Build history of the part. All positions in model axes, mm. A direction names the side the tool comes from. Give positions to 0.01 mm unless a question says otherwise; leave off trailing zeros. Loops run counter-clockwise (first coordinate to the right, second up) from the corner with the lowest first, then second, coordinate; pieces in that order, holes last.
1) Band-saw the part on C-C on x = 19. List the corners of the cut face in (y, z).
2) Band-saw the part on D-D on y = 39. List the corners of the cut face in (x, z), then the cut area to 3 significant figures.
3) 3-axis set-ups, long thin cutter, end or side, ignore diameter. For faces 1 (the flat face through (-21, 10, 0)), 2 (the flat face through (0, 21, 0)), 3 (the flat face through (-4.93, 28.9, -8.7)), 4 (the flat face through (-10, 29, 0)): which of +Z, -Z, +X, -X, +Y, -Y reach the whole face in a straight line?
4) Wall check: line 1 (X direction, y = 12.3, z = -20); line 2 (X direction, y = 13, z = 0). Give the ranges that are in metal, low to high.
5) Band-saw the part on B-B on z = 0. List the corners of the cut face in (x, y), then the cut area to 3 significant figures.
6) Flat gauge pins, fed straight in: P1, Ø1.5, axis at x = -4, y = 24, coming from the -Z side; P2, Ø22.5, axis at x = 5, z = 4.5, coming from the -Y side; P3, Ø3, axis at y = 40.5, z = -6.5, coming from the -X side (3 decimals); P4, Ø3, axis at y = 40.5, z = 10, coming from the -X side. Where does each tip first touch, or does it go through?
7) Band-saw the part on A-A on y = 5.5. List the corners of the cut face in (x, z), then the cut area to 3 significant figures.
8) Two-plate mould, pull along Z, no slides. Class faces 5 (the flat face through (0, 10, 21)), 6 (the cylindrical face through (-26.68, 4.93, -0.3)), 7 (the cylindrical face through (-25.68, 4.44, -0.29)): +Z half, -Z half, draft (parallel to the pull), parting line (faces both ways), or undercut.
```python
from build123d import *

# Parameters (mm, degrees)
SKETCH3_R             = 4
BOSS_EXTRUDE2_DEPTH   = 10
SKETCH4_R             = 15
BOSS_EXTRUDE3_DEPTH   = 12
SHELL2_T              = -1
BOSS_EXTRUDE4_DEPTH   = 14
SKETCH6_R             = 8
BOSS_EXTRUDE5_DEPTH   = 12
BOSS_EXTRUDE6_DEPTH   = 5
M5X0_8_TAPPED_HOLE1_D = 4.2


with BuildPart() as part:
    # Sketch3 → Boss-Extrude2 (new body)
    with BuildSketch(Plane(origin=(0, 0, 0), x_dir=(1, 0, 0), z_dir=(0, 1, 0))):
        with Locations((-20, -20)):
            Circle(SKETCH3_R)
        with BuildLine():
            ThreePointArc((23.859011112, 21.052631579), (23.964596098, 20.531015797), (24, 20))
            ThreePointArc((24, 20), (16.821122343, 17.572092085), (21.052631579, 23.859011112))
            ThreePointArc((21.052631579, 23.859011112), (0, 26.678788881), (-21.052631579, 23.859011112))
            ThreePointArc((-21.052631579, 23.859011112), (-17.572092085, 23.178877657), (-16, 20))
            ThreePointArc((-16, 20), (-20.531015797, 16.035403902), (-23.859011112, 21.052631579))
            ThreePointArc((-23.859011112, 21.052631579), (-26.678788881, 0), (-23.859011112, -21.052631579))
            ThreePointArc((-23.859011112, -21.052631579), (-20.531015797, -16.035403902), (-16, -20))
            ThreePointArc((-16, -20), (-17.572092085, -23.178877657), (-21.052631579, -23.859011112))
            ThreePointArc((-21.052631579, -23.859011112), (0, -26.678788881), (21.052631579, -23.859011112))
            ThreePointArc((21.052631579, -23.859011112), (16.821122343, -17.572092085), (24, -20))
            ThreePointArc((24, -20), (23.964596098, -20.531015797), (23.859011112, -21.052631579))
            ThreePointArc((23.859011112, -21.052631579), (26.678788881, 0), (23.859011112, 21.052631579))
        make_face()
        with Locations((-20, 20)):
            Circle(SKETCH3_R)
        with Locations((20, -20)):
            Circle(SKETCH3_R)
        with Locations((20, 20)):
            Circle(SKETCH3_R)
    extrude(amount=BOSS_EXTRUDE2_DEPTH)

    # Sketch4 → Boss-Extrude3 (add)
    with BuildSketch(Plane(origin=(0, 10, 0), x_dir=(1, 0, 0), z_dir=(0, 1, 0))):
        with Locations(Location((0, 0, 0), (0, 0, 270))):
            Circle(SKETCH4_R)
    extrude(amount=BOSS_EXTRUDE3_DEPTH)

    # Shell2
    shell2_openings = [part.faces().sort_by_distance(p)[0] for p in [
        (0, 0, 0),
    ]]
    offset(amount=SHELL2_T, openings=shell2_openings, kind=Kind.INTERSECTION)

    # Sketch5 → Boss-Extrude4 (add)
    with BuildSketch(Plane(origin=(0, 22, 0), x_dir=(1, 0, 0), z_dir=(0, 1, 0))):
        Polygon((0, 11.547005384), (-10, 5.773502692), (-10, -5.773502692), (0, -11.547005384), (10, -5.773502692), (10, 5.773502692), align=None)
    extrude(amount=BOSS_EXTRUDE4_DEPTH)

    # Sketch6 → Boss-Extrude5 (add)
    with BuildSketch(Plane(origin=(0, 36, 0), x_dir=(1, 0, 0), z_dir=(0, 1, 0))):
        with Locations(Location((0, 0, 0), (0, 0, 270))):
            Circle(SKETCH6_R)
    extrude(amount=BOSS_EXTRUDE5_DEPTH)

    # Sketch7 → Boss-Extrude6 (add)
    with BuildSketch(Plane(origin=(0, 10, 0), x_dir=(1, 0, 0), z_dir=(0, 1, 0))):
        with BuildLine():
            ThreePointArc((23.859011112, 21.052631579), (22.828427125, 22.828427125), (21.052631579, 23.859011112))
            ThreePointArc((21.052631579, 23.859011112), (18.973409384, 23.866020138), (17.171572875, 22.828427125))
            ThreePointArc((17.171572875, 22.828427125), (16.30448187, 21.530733729), (16, 20))
            Line((16, 20), (20, 20))
            Line((20, 20), (20, 16))
            ThreePointArc((20, 16), (21.530733729, 16.30448187), (22.828427125, 17.171572875))
            ThreePointArc((22.828427125, 17.171572875), (23.69551813, 18.469266271), (24, 20))
            ThreePointArc((24, 20), (23.964596098, 20.531015797), (23.859011112, 21.052631579))
        make_face()
        with BuildLine():
            Line((20, 20), (16, 20))
            ThreePointArc((16, 20), (16.30448187, 18.469266271), (17.171572875, 17.171572875))
            Line((17.171572875, 17.171572875), (20, 20))
        make_face()
        with BuildLine():
            Line((20, 16), (20, 20))
            Line((20, 20), (17.171572875, 17.171572875))
            ThreePointArc((17.171572875, 17.171572875), (18.469266271, 16.30448187), (20, 16))
        make_face()
        with BuildLine():
            Line((17.171572875, 17.171572875), (10.606601718, 10.606601718))
            ThreePointArc((10.606601718, 10.606601718), (11.937336386, 9.082951062), (13.050951275, 7.394097025))
            Line((13.050951275, 7.394097025), (20, 14.343145751))
            Line((20, 14.343145751), (20, 16))
            ThreePointArc((20, 16), (18.469266271, 16.30448187), (17.171572875, 17.171572875))
        make_face()
        with BuildLine():
            Line((16, 20), (14.343145751, 20))
            Line((14.343145751, 20), (7.394097025, 13.050951275))
            ThreePointArc((7.394097025, 13.050951275), (9.082951062, 11.937336386), (10.606601718, 10.606601718))
            Line((10.606601718, 10.606601718), (17.171572875, 17.171572875))
            ThreePointArc((17.171572875, 17.171572875), (16.30448187, 18.469266271), (16, 20))
        make_face()
        with BuildLine():
            ThreePointArc((-7.394097025, -13.050951275), (-9.082951062, -11.937336386), (-10.606601718, -10.606601718))
            Line((-10.606601718, -10.606601718), (-17.171572875, -17.171572875))
            ThreePointArc((-17.171572875, -17.171572875), (-16.30448187, -18.469266271), (-16, -20))
            Line((-16, -20), (-14.343145751, -20))
            Line((-14.343145751, -20), (-7.394097025, -13.050951275))
        make_face()
        with BuildLine():
            Line((-17.171572875, -17.171572875), (-10.606601718, -10.606601718))
            ThreePointArc((-10.606601718, -10.606601718), (-11.937336386, -9.082951062), (-13.050951275, -7.394097025))
            Line((-13.050951275, -7.394097025), (-20, -14.343145751))
            Line((-20, -14.343145751), (-20, -16))
            ThreePointArc((-20, -16), (-18.469266271, -16.30448187), (-17.171572875, -17.171572875))
        make_face()
        with BuildLine():
            ThreePointArc((-16, -20), (-16.30448187, -18.469266271), (-17.171572875, -17.171572875))
            Line((-17.171572875, -17.171572875), (-20, -20))
            Line((-20, -20), (-16, -20))
        make_face()
        with BuildLine():
            Line((-20, -20), (-17.171572875, -17.171572875))
            ThreePointArc((-17.171572875, -17.171572875), (-18.469266271, -16.30448187), (-20, -16))
            Line((-20, -16), (-20, -20))
        make_face()
        with BuildLine():
            ThreePointArc((-22.828427125, -17.171572875), (-23.866020138, -18.973409384), (-23.859011112, -21.052631579))
            ThreePointArc((-23.859011112, -21.052631579), (-22.828427125, -22.828427125), (-21.052631579, -23.859011112))
            ThreePointArc((-21.052631579, -23.859011112), (-18.973409384, -23.866020138), (-17.171572875, -22.828427125))
            ThreePointArc((-17.171572875, -22.828427125), (-16.30448187, -21.530733729), (-16, -20))
            Line((-16, -20), (-20, -20))
            Line((-20, -20), (-20, -16))
            ThreePointArc((-20, -16), (-21.530733729, -16.30448187), (-22.828427125, -17.171572875))
        make_face()
        with BuildLine():
            ThreePointArc((21.052631579, -23.859011112), (22.828427125, -22.828427125), (23.859011112, -21.052631579))
            ThreePointArc((23.859011112, -21.052631579), (23.964596098, -20.531015797), (24, -20))
            ThreePointArc((24, -20), (23.69551813, -18.469266271), (22.828427125, -17.171572875))
            ThreePointArc((22.828427125, -17.171572875), (21.530733729, -16.30448187), (20, -16))
            Line((20, -16), (20, -20))
            Line((20, -20), (16, -20))
            ThreePointArc((16, -20), (16.30448187, -21.530733729), (17.171572875, -22.828427125))
            ThreePointArc((17.171572875, -22.828427125), (18.973409384, -23.866020138), (21.052631579, -23.859011112))
        make_face()
        with BuildLine():
            Line((20, -20), (17.171572875, -17.171572875))
            ThreePointArc((17.171572875, -17.171572875), (16.30448187, -18.469266271), (16, -20))
            Line((16, -20), (20, -20))
        make_face()
        with BuildLine():
            ThreePointArc((20, -16), (18.469266271, -16.30448187), (17.171572875, -17.171572875))
            Line((17.171572875, -17.171572875), (20, -20))
            Line((20, -20), (20, -16))
        make_face()
        with BuildLine():
            ThreePointArc((13.050951275, -7.394097025), (11.937336386, -9.082951062), (10.606601718, -10.606601718))
            Line((10.606601718, -10.606601718), (17.171572875, -17.171572875))
            ThreePointArc((17.171572875, -17.171572875), (18.469266271, -16.30448187), (20, -16))
            Line((20, -16), (20, -14.343145751))
            Line((20, -14.343145751), (13.050951275, -7.394097025))
        make_face()
        with BuildLine():
            Line((17.171572875, -17.171572875), (10.606601718, -10.606601718))
            ThreePointArc((10.606601718, -10.606601718), (9.082951062, -11.937336386), (7.394097025, -13.050951275))
            Line((7.394097025, -13.050951275), (14.343145751, -20))
            Line((14.343145751, -20), (16, -20))
            ThreePointArc((16, -20), (16.30448187, -18.469266271), (17.171572875, -17.171572875))
        make_face()
        with BuildLine():
            Line((17.171572875, 22.828427125), (14.343145751, 20))
            Line((14.343145751, 20), (16, 20))
            ThreePointArc((16, 20), (16.30448187, 21.530733729), (17.171572875, 22.828427125))
        make_face()
        with BuildLine():
            ThreePointArc((22.828427125, 17.171572875), (21.530733729, 16.30448187), (20, 16))
            Line((20, 16), (20, 14.343145751))
            Line((20, 14.343145751), (22.828427125, 17.171572875))
        make_face()
        with BuildLine():
            ThreePointArc((-16, 20), (-16.30448187, 21.530733729), (-17.171572875, 22.828427125))
            ThreePointArc((-17.171572875, 22.828427125), (-18.973409384, 23.866020138), (-21.052631579, 23.859011112))
            ThreePointArc((-21.052631579, 23.859011112), (-22.828427125, 22.828427125), (-23.859011112, 21.052631579))
            ThreePointArc((-23.859011112, 21.052631579), (-23.866020138, 18.973409384), (-22.828427125, 17.171572875))
            ThreePointArc((-22.828427125, 17.171572875), (-21.530733729, 16.30448187), (-20, 16))
            Line((-20, 16), (-20, 20))
            Line((-20, 20), (-16, 20))
        make_face()
        with BuildLine():
            Line((-20, 14.343145751), (-20, 16))
            ThreePointArc((-20, 16), (-21.530733729, 16.30448187), (-22.828427125, 17.171572875))
            Line((-22.828427125, 17.171572875), (-20, 14.343145751))
        make_face()
        with BuildLine():
            Line((-17.171572875, 17.171572875), (-20, 20))
            Line((-20, 20), (-20, 16))
            ThreePointArc((-20, 16), (-18.469266271, 16.30448187), (-17.171572875, 17.171572875))
        make_face()
        with BuildLine():
            ThreePointArc((-17.171572875, 17.171572875), (-16.30448187, 18.469266271), (-16, 20))
            Line((-16, 20), (-20, 20))
            Line((-20, 20), (-17.171572875, 17.171572875))
        make_face()
        with BuildLine():
            Line((-14.343145751, 20), (-17.171572875, 22.828427125))
            ThreePointArc((-17.171572875, 22.828427125), (-16.30448187, 21.530733729), (-16, 20))
            Line((-16, 20), (-14.343145751, 20))
        make_face()
        with BuildLine():
            Line((-7.394097025, 13.050951275), (-14.343145751, 20))
            Line((-14.343145751, 20), (-16, 20))
            ThreePointArc((-16, 20), (-16.30448187, 18.469266271), (-17.171572875, 17.171572875))
            Line((-17.171572875, 17.171572875), (-10.606601718, 10.606601718))
            ThreePointArc((-10.606601718, 10.606601718), (-9.082951062, 11.937336386), (-7.394097025, 13.050951275))
        make_face()
        with BuildLine():
            Line((-10.606601718, 10.606601718), (-17.171572875, 17.171572875))
            ThreePointArc((-17.171572875, 17.171572875), (-18.469266271, 16.30448187), (-20, 16))
            Line((-20, 16), (-20, 14.343145751))
            Line((-20, 14.343145751), (-13.050951275, 7.394097025))
            ThreePointArc((-13.050951275, 7.394097025), (-11.937336386, 9.082951062), (-10.606601718, 10.606601718))
        make_face()
        with BuildLine():
            ThreePointArc((-16, -20), (-16.30448187, -21.530733729), (-17.171572875, -22.828427125))
            Line((-17.171572875, -22.828427125), (-14.343145751, -20))
            Line((-14.343145751, -20), (-16, -20))
        make_face()
        with BuildLine():
            Line((-20, -16), (-20, -14.343145751))
            Line((-20, -14.343145751), (-22.828427125, -17.171572875))
            ThreePointArc((-22.828427125, -17.171572875), (-21.530733729, -16.30448187), (-20, -16))
        make_face()
        with BuildLine():
            Line((16, -20), (14.343145751, -20))
            Line((14.343145751, -20), (17.171572875, -22.828427125))
            ThreePointArc((17.171572875, -22.828427125), (16.30448187, -21.530733729), (16, -20))
        make_face()
        with BuildLine():
            Line((22.828427125, -17.171572875), (20, -14.343145751))
            Line((20, -14.343145751), (20, -16))
            ThreePointArc((20, -16), (21.530733729, -16.30448187), (22.828427125, -17.171572875))
        make_face()
    extrude(amount=BOSS_EXTRUDE6_DEPTH)

    # M5x0.8 Tapped Hole1 (through all)
    with Locations(Plane(origin=(0, 15, 0), x_dir=(1, 0, 0), z_dir=(0, 1, 0))):
        with Locations((20, -20), (20, 20), (-20, 20), (-20, -20)):
            Hole(M5X0_8_TAPPED_HOLE1_D / 2)


solid = part.part
```
Findings below:
1. outline: (0, -24.39) - (10, -24.39) - (10, -23.87) - (15, -23.87) - (15, -21.85) - (9, -21.85) - (9, -23.36) - (0, -23.36) - close; (0, 23.36) - (9, 23.36) - (9, 21.85) - (15, 21.85) - (15, 23.87) - (10, 23.87) - (10, 24.39) - (0, 24.39) - close; (9, -18.15) - (15, -18.15) - (15, -13.34) - (10, -13.34) - (10, 13.34) - (15, 13.34) - (15, 18.15) - (9, 18.15) - close
2. outline: circle Ø16 at (0, 0)
2. area: 201 mm2
3. face 1: -X, +Y
3. face 2: -Y
3. face 3: -Z, -X, +Y
3. face 4: +Z, -Z, -X, +Y
4. line 1: x = -24 to -22.1, -17.9 to -14.34, 14.34 to 17.9, 22.1 to 24
4. line 2: x = -15 to -14, 14 to 15
5. outline: (-26.68, 0) - (-25.68, 0) - (-25.68, 9) - (-14, 9) - (-14, 21) - (14, 21) - (14, 9) - (25.68, 9) - (25.68, 0) - (26.68, 0) - (26.68, 10) - (15, 10) - (15, 22) - (10, 22) - (10, 36) - (8, 36) - (8, 48) - (-8, 48) - (-8, 36) - (-10, 36) - (-10, 22) - (-15, 22) - (-15, 10) - (-26.68, 10) - close
5. area: 567 mm2
6. P1: stops at z = -9.67
6. P2: stops at y = 9
6. P3: stops at x = -6.245
6. P4: passes through
7. outline: (-23.86, -21.05) arc R4 ccw to (-21.05, -23.86) arc R80 ccw to (21.05, -23.86) arc R4 ccw to (23.86, -21.05) arc R80 ccw to (23.86, 21.05) arc R4 ccw to (21.05, 23.86) arc R80 ccw to (-21.05, 23.86) arc R4 ccw to (-23.86, 21.05) arc R80 ccw to start; hole (-22.89, -20.79) arc R3 ccw to (-20.79, -22.89) arc R79 ccw to (20.79, -22.89) arc R3 ccw to (22.89, -20.79) arc R79 ccw to (22.89, 20.79) arc R3 ccw to (20.79, 22.89) arc R79 ccw to (-20.79, 22.89) arc R3 ccw to (-22.89, 20.79) arc R79 ccw to start
7. area: 184 mm2
8. face 5: draft
8. face 6: parting line
8. face 7: undercut
